Design review of the part shown in the three views and the two pictorial views. Dimensions are in mm from the part's minimum x, y and z. A direction names the side the tool comes from. Round coordinates to 2 decimals unless told otherwise and drop trailing zeros. Write each loop counter-clockwise with the first axis right and the second up, starting at its lowest first coordinate (ties: lowest second). Pieces come first, ordered by that corner, then holes. Notation, with made-up numbers: (45.25, 15.5) -> (73.25, 15.5) arc R23 cw to (73.25, 28.5) -> close; hole circle Ø2 at (-5.5, -30.75). An arc over 180 degrees is marked (long way). Answer as a JSON object with one key per item and string values. Group by question number.
1) We need section B-B, the plane y = 10.25. Write out the cut boundary in (x, z) (1 decimal).
2) Machinability: for the marked faces 1 and 2, which of the approach directions +Z, -Z, +X, -X, +Y, -Y give a long, thin tool a straight path to every point of the face, cutting with its end or side? Answer none if there is none.
3) We need section D-D, the plane z = 10. Write out the cut boundary in (x, y), then the cut area to 3 significant figures.
4) To check wall thickness, follow probe 1 along Y at (x, z) = (72.5, 67); probe 2 along Z at (x, y) = (41.5, 1.75) (1 decimal); probe 3 along Z at (x, y) = (72.5, 9) (1 decimal). State the ranges of each line that lie inside material, in increasing order. Write a range as [from, to].
5) We need section C-C, the plane x = 10. Write out the cut boundary in (y, z).
6) Insertion check: pin 1 Ø2.5 at (x, y) = (38, 8.5) entering from +Z; pin 2 Ø6 at (x, y) = (15.5, 5) entering from +Z; pin 3 Ø4 at (x, y) = (38, 6.5) entering from -Z; pin 4 Ø8 at (x, z) = (59, 32.5) entering from +Y. Each pin has a flat end and moves straight along its axis. Give the tip position at first contact, or say it passes through.
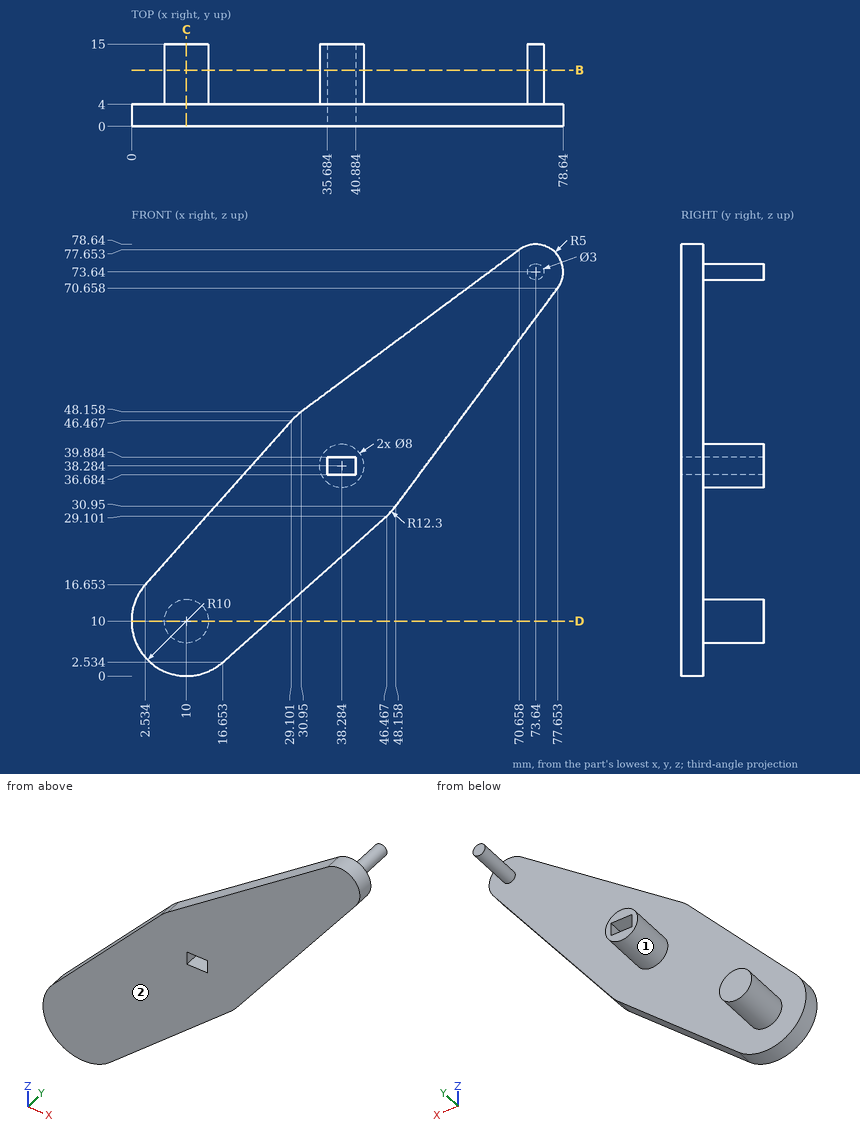
Here are the results:
{
 "1": {"outline": "circle Ø8 at (10, 10); circle Ø8 at (38.3, 38.3); circle Ø3 at (73.6, 73.6); hole (35.7, 36.7) -> (40.9, 36.7) -> (40.9, 39.9) -> (35.7, 39.9) -> close"},
 "2": {"face 1": "+Y", "face 2": "+Z, -Z, +X, -X, -Y"},
 "3": {"outline": "(0, 0) -> (25.03, 0) -> (25.03, 4) -> (14, 4) -> (14, 15) -> (6, 15) -> (6, 4) -> (0, 4) -> close", "area": "188 mm^2"},
 "4": {"probe 1": "y = [0, 4]", "probe 2": "z = [24.7, 56]", "probe 3": "z = [72.7, 74.6]"},
 "5": {"outline": "(0, 0) -> (4, 0) -> (4, 6) -> (15, 6) -> (15, 14) -> (4, 14) -> (4, 25.03) -> (0, 25.03) -> close"},
 "6": {"pin 1": "stops at z = 42.28", "pin 2": "stops at z = 34.38", "pin 3": "stops at z = 34.28", "pin 4": "passes through"}
}
